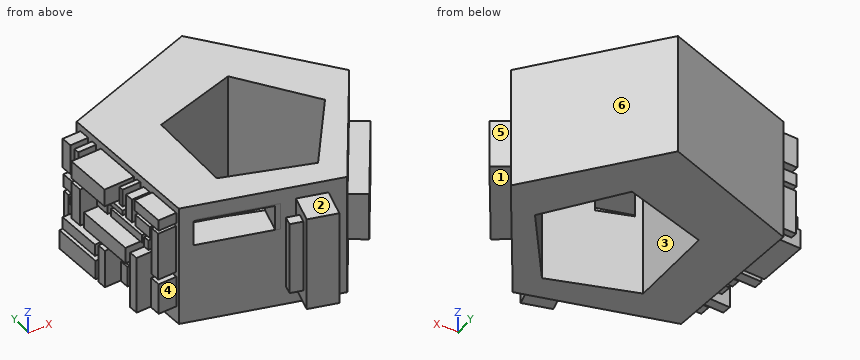
```python
from build123d import *

# Parameters (mm, degrees)
F1_DEPTH  = 25.4
F2_DEPTH  = 25.4
F3_W      = 42.2709332779
F3_H      = 19.9366761371
F4_DEPTH  = 7.62
F5_W      = 11.9896456599
F5_H      = 39.5106691867
F6_DEPTH  = 12.7
F7_W      = 31.212631613
F7_H      = 11.2281162292
F8_DEPTH  = 7.62
F9_W      = 29.9386493862
F9_H      = 10.5491885915
F10_DEPTH = 12.7
F11_W     = 4.0996596217
F11_H     = 30.3628398106
F12_DEPTH = 5.08
F13_W     = 20.0984636322
F13_H     = 7.4342815205
F13_W_2   = 5.3358711302
F13_H_2   = 15.8698209561
F13_W_3   = 25.2564756665
F13_H_3   = 6.7615092266
F13_W_4   = 3.9129797369
F13_H_4   = 16.0269849002
F13_W_5   = 19.5648819208
F13_H_5   = 4.9852463417
F13_W_6   = 21.8770895153
F13_H_6   = 8.1112636253
F13_W_7   = 3.8565089926
F13_H_7   = 24.0716314875
F14_DEPTH = 12.7
F15_W     = 2.3439750075
F15_H     = 14.3474126235
F15_W_2   = 10.4969404638
F15_H_2   = 5.3929993883
F15_W_3   = 4.6879537404
F15_H_3   = 12.7176120877
F15_W_4   = 2.7516260743
F15_H_4   = 18.800791353
F15_W_5   = 6.8281069398
F15_H_5   = 3.639341332
F15_W_6   = 10.8026759699
F15_H_6   = 4.3754521757
F15_W_7   = 4.6879523434
F15_H_7   = 8.343886584
F15_W_8   = 3.7707453594
F15_H_8   = 8.649148047
F15_W_9   = 6.2166322023
F15_H_9   = 3.6631692201
F15_W_10  = 14.7772468626
F15_H_10  = 2.1284492686
F15_W_11  = 18.8184157014
F15_H_11  = 3.3579049632
F15_W_12  = 3.6688325927
F15_H_12  = 10.0737148896
F15_W_13  = 1.9363295287
F15_H_13  = 7.4342815205
F15_W_14  = 14.4715099595
F15_H_14  = 4.57723625
F15_W_15  = 8.7644355372
F15_H_15  = 4.8842262477
F15_W_16  = 3.9745708928
F15_H_16  = 20.249187015
F15_W_17  = 2.5478007738
F15_H_17  = 4.1719428264
F15_W_18  = 4.586043302
F15_H_18  = 13.0246016197
F16_DEPTH = 7.62
F17_W     = 61.8985138723
F17_H     = 50.8
F17_W_2   = 21.8770895153
F17_H_2   = 8.1112636253
F17_W_3   = 2.7516260743
F17_H_3   = 18.800791353
F17_W_4   = 6.8281069398
F17_H_4   = 3.639341332
F17_W_5   = 19.5648819208
F17_H_5   = 4.9852463417
F17_W_6   = 3.7707453594
F17_H_6   = 8.649148047
F17_W_7   = 4.6879523434
F17_H_7   = 8.343886584
F17_W_8   = 3.9129797369
F17_H_8   = 16.0269849002
F17_W_9   = 10.8026759699
F17_H_9   = 4.3754521757
F17_W_10  = 3.8565089926
F17_H_10  = 24.0716314875
F17_W_11  = 4.586043302
F17_H_11  = 13.0246016197
F17_W_12  = 10.4969404638
F17_H_12  = 5.3929993883
F17_W_13  = 5.3358711302
F17_H_13  = 15.8698209561
F17_W_14  = 6.2166322023
F17_H_14  = 3.6631692201
F17_W_15  = 4.6879537404
F17_H_15  = 12.7176120877
F17_W_16  = 2.3439750075
F17_H_16  = 14.3474126235
F17_W_17  = 20.0984636322
F17_H_17  = 7.4342815205
F17_W_18  = 25.2564756665
F17_H_18  = 6.7615092266
F17_W_19  = 14.7772468626
F17_H_19  = 2.1284492686
F17_W_20  = 18.8184157014
F17_H_20  = 3.3579049632
F17_W_21  = 2.5478007738
F17_H_21  = 4.1719428264
F17_W_22  = 3.9745708928
F17_H_22  = 20.249187015
F17_W_23  = 1.9363295287
F17_W_24  = 3.6688325927
F17_H_23  = 10.0737148896
F17_W_25  = 8.7644355372
F17_H_24  = 4.8842262477
F17_W_26  = 14.4715099595
F17_H_25  = 4.57723625
F18_DEPTH = 5.08
F20_DEPTH = 76.2
F21_DEPTH = 5.08


with BuildPart() as f1:
    # F0 (on Top) → F1 (new body)
    with BuildSketch(Plane.XY):
        Polygon((-16.7726497146, -31.6705114622), (16.7726497146, 20.3500508744), (-22.335777472, 68.3287643065), (-80.051414149, 45.9606776074), (-76.6132121111, -15.842273668), align=None)
    extrude(amount=F1_DEPTH)

    # F2 (add): a face of the model
    f2_faces = [f1.faces().sort_by_distance(p)[0] for p in [
        (-35.8000807464, 17.4253415316, 0),
    ]]
    extrude(f2_faces, amount=F2_DEPTH)

    # F3 (on face) → F4 (join)
    with BuildSketch(Plane(origin=(2.5779849193, -1.6624056365, 0), x_dir=(0.5419403041, 0.8404169839, 0), z_dir=(0.8404169839, -0.5419403041, 0))):
        with Locations((-5.966336932, 1.3790032826)):
            Rectangle(F3_W, F3_H)
    extrude(amount=F4_DEPTH)

    # F5 (on face) → F6 (join)
    with BuildSketch(Plane(origin=(-8.9260455296, -33.7459919046, 0), x_dir=(0.9667528128, -0.2557127272, 0), z_dir=(-0.2557127272, -0.9667528128, 0))):
        with Locations((-20.9904853255, 0.3661895171)):
            Rectangle(F5_W, F5_H)
    extrude(amount=F6_DEPTH)

    # F7 (on face) → F8 (join)
    with BuildSketch(Plane(origin=(-8.9260455296, -33.7459919046, 0), x_dir=(0.9667528128, -0.2557127272, 0), z_dir=(-0.2557127272, -0.9667528128, 0))):
        with Locations((-48.2821147889, 13.5751133785)):
            Rectangle(F7_W, F7_H)
    extrude(amount=-F8_DEPTH)

    # F9 (on face) → F10 (cut)
    with BuildSketch(Plane(origin=(-8.9260455296, -33.7459919046, 0), x_dir=(0.9667528128, -0.2557127272, 0), z_dir=(-0.2557127272, -0.9667528128, 0))):
        with Locations((-49.556100741, 13.31924228)):
            Rectangle(F9_W, F9_H)
    extrude(amount=-F10_DEPTH, mode=Mode.SUBTRACT)

    # F11 (on face) → F12 (join)
    with BuildSketch(Plane(origin=(-26.0881225645, 6.9004867437, 0), x_dir=(-0.2557127272, -0.9667528128, 0), z_dir=(-0.9667528128, 0.2557127272, 0))):
        with Locations((41.5847562253, 1.0980186053)):
            Rectangle(F11_W, F11_H)
    extrude(amount=F12_DEPTH)

    # F13 (on face) → F14 (join)
    with BuildSketch(Plane(origin=(-77.2554477784, -4.2978503859, 0), x_dir=(0.055545793, -0.9984561407, 0), z_dir=(-0.9984561407, -0.055545793, 0))):
        with Locations((-25.5797388963, 18.8945052214)):
            Rectangle(F13_W, F13_H)
        with Locations((-32.961031422, 5.5121385958)):
            Rectangle(F13_W_2, F13_H_2)
        with Locations((-15.5305069638, 1.3388268417)):
            Rectangle(F13_W_3, F13_H_3)
        with Locations((-17.3091338947, -12.3113878071)):
            Rectangle(F13_W_4, F13_H_4)
        with Locations((-31.1824083328, -7.7815449331)):
            Rectangle(F13_W_5, F13_H_5)
        with Locations((-31.9827897474, -16.2692484446)):
            Rectangle(F13_W_6, F13_H_6)
        with Locations((1.9282544963, -7.5779159088)):
            Rectangle(F13_W_7, F13_H_7)
    extrude(amount=F14_DEPTH)

    # F15 (on face) → F16 (join)
    with BuildSketch(Plane(origin=(-77.2554477784, -4.2978503859, 0), x_dir=(0.055545793, -0.9984561407, 0), z_dir=(-0.9984561407, -0.055545793, 0))):
        with Locations((-39.761338383, 15.3379100375)):
            Rectangle(F15_W, F15_H)
        with Locations((-42.4110535532, 4.5519121923)):
            Rectangle(F15_W_2, F15_H_2)
        with Locations((-45.7231942564, 16.2528399378)):
            Rectangle(F15_W_3, F15_H_3)
        with Locations((-45.9779724479, -9.4003956765)):
            Rectangle(F15_W_4, F15_H_4)
        with Locations((-39.9651639163, -1.819670666)):
            Rectangle(F15_W_5, F15_H_5)
        with Locations((-7.5061791576, -6.2340861186)):
            Rectangle(F15_W_6, F15_H_6)
        with Locations((-4.7545537818, -13.407792896)):
            Rectangle(F15_W_7, F15_H_7)
        with Locations((-10.7164080255, -13.8656888157)):
            Rectangle(F15_W_8, F15_H_8)
        with Locations((-24.066885002, 8.0624492839)):
            Rectangle(F15_W_9, F15_H_9)
        with Locations((-19.1751066595, 12.3828244396)):
            Rectangle(F15_W_10, F15_H_10)
        with Locations((-9.4092078507, 8.2150814123)):
            Rectangle(F15_W_11, F15_H_11)
        with Locations((-7.9138264991, 16.7624759488)):
            Rectangle(F15_W_12, F15_H_12)
        with Locations((-12.7546479926, 18.8945052214)):
            Rectangle(F15_W_13, F15_H_13)
        with Locations((2.7869374026, 20.3230278566)):
            Rectangle(F15_W_14, F15_H_14)
        with Locations((0.3410479985, 13.9642218128)):
            Rectangle(F15_W_15, F15_H_15)
        with Locations((7.8315832652, 6.4852521755)):
            Rectangle(F15_W_16, F15_H_16)
        with Locations((2.5321574649, 7.8080624808)):
            Rectangle(F15_W_17, F15_H_17)
        with Locations((7.831583498, -11.9832272176)):
            Rectangle(F15_W_18, F15_H_18)
    extrude(amount=F16_DEPTH)

    # F17 (on face) → F18 (cut)
    with BuildSketch(Plane(origin=(-77.2554477784, -4.2978503859, 0), x_dir=(0.055545793, -0.9984561407, 0), z_dir=(-0.9984561407, -0.055545793, 0))):
        with Locations((-19.38698313, 0)):
            Rectangle(F17_W, F17_H)
        with Locations((-31.9827897474, -16.2692484446)):
            Rectangle(F17_W_2, F17_H_2, mode=Mode.SUBTRACT)
        with Locations((-45.9779724479, -9.4003956765)):
            Rectangle(F17_W_3, F17_H_3, mode=Mode.SUBTRACT)
        with Locations((-39.9651639163, -1.819670666)):
            Rectangle(F17_W_4, F17_H_4, mode=Mode.SUBTRACT)
        with Locations((-31.1824083328, -7.7815449331)):
            Rectangle(F17_W_5, F17_H_5, mode=Mode.SUBTRACT)
        with Locations((-10.7164080255, -13.8656888157)):
            Rectangle(F17_W_6, F17_H_6, mode=Mode.SUBTRACT)
        with Locations((-4.7545537818, -13.407792896)):
            Rectangle(F17_W_7, F17_H_7, mode=Mode.SUBTRACT)
        with Locations((-17.3091338947, -12.3113878071)):
            Rectangle(F17_W_8, F17_H_8, mode=Mode.SUBTRACT)
        with Locations((-7.5061791576, -6.2340861186)):
            Rectangle(F17_W_9, F17_H_9, mode=Mode.SUBTRACT)
        with Locations((1.9282544963, -7.5779159088)):
            Rectangle(F17_W_10, F17_H_10, mode=Mode.SUBTRACT)
        with Locations((7.831583498, -11.9832272176)):
            Rectangle(F17_W_11, F17_H_11, mode=Mode.SUBTRACT)
        with Locations((-42.4110535532, 4.5519121923)):
            Rectangle(F17_W_12, F17_H_12, mode=Mode.SUBTRACT)
        with Locations((-32.961031422, 5.5121385958)):
            Rectangle(F17_W_13, F17_H_13, mode=Mode.SUBTRACT)
        with Locations((-24.066885002, 8.0624492839)):
            Rectangle(F17_W_14, F17_H_14, mode=Mode.SUBTRACT)
        with Locations((-45.7231942564, 16.2528399378)):
            Rectangle(F17_W_15, F17_H_15, mode=Mode.SUBTRACT)
        with Locations((-39.761338383, 15.3379100375)):
            Rectangle(F17_W_16, F17_H_16, mode=Mode.SUBTRACT)
        with Locations((-25.5797388963, 18.8945052214)):
            Rectangle(F17_W_17, F17_H_17, mode=Mode.SUBTRACT)
        with Locations((-15.5305069638, 1.3388268417)):
            Rectangle(F17_W_18, F17_H_18, mode=Mode.SUBTRACT)
        with Locations((-19.1751066595, 12.3828244396)):
            Rectangle(F17_W_19, F17_H_19, mode=Mode.SUBTRACT)
        with Locations((-9.4092078507, 8.2150814123)):
            Rectangle(F17_W_20, F17_H_20, mode=Mode.SUBTRACT)
        with Locations((2.5321574649, 7.8080624808)):
            Rectangle(F17_W_21, F17_H_21, mode=Mode.SUBTRACT)
        with Locations((7.8315832652, 6.4852521755)):
            Rectangle(F17_W_22, F17_H_22, mode=Mode.SUBTRACT)
        with Locations((-12.7546479926, 18.8945052214)):
            Rectangle(F17_W_23, F17_H_17, mode=Mode.SUBTRACT)
        with Locations((-7.9138264991, 16.7624759488)):
            Rectangle(F17_W_24, F17_H_23, mode=Mode.SUBTRACT)
        with Locations((0.3410479985, 13.9642218128)):
            Rectangle(F17_W_25, F17_H_24, mode=Mode.SUBTRACT)
        with Locations((2.7869374026, 20.3230278566)):
            Rectangle(F17_W_26, F17_H_25, mode=Mode.SUBTRACT)
    extrude(amount=-F18_DEPTH, mode=Mode.SUBTRACT)

    # F19 (on face) → F20 (cut)
    with BuildSketch(Plane.XY.offset(25.4)):
        Polygon((-55.9489503503, 28.6254710477), (-55.9489503503, -8.0040893477), (-21.1121682472, -19.3232460063), (0.4181471511, 10.31069085), (-21.1121682472, 39.9446277064), align=None)
    extrude(amount=-F20_DEPTH, mode=Mode.SUBTRACT)

    # F21 (add): a face of the model
    f21_faces = [f1.faces().sort_by_distance(p)[0] for p in [
        (-71.5855334196, -14.7605835197, 0),
    ]]
    extrude(f21_faces, amount=F21_DEPTH)


solid = f1.part
```
Here's how the part is built. I have some questions about the finished solid (model axes, mm). Face numbers are marked on the shaded views. A direction names the side the tool comes from. Give positions to 0.01 mm unless a question says otherwise; leave off trailing zeros. Write each loop counter-clockwise with the first axis right and the second up, starting at its lowest first coordinate (ties: lowest second). Pieces come first, ordered by that corner, then holes. Notation, with made-up numbers: (68.25, 25) -> (79.25, 25) arc R25 cw to (79.25, 61) -> close; hole circle Ø8 at (43.25, 31). An arc over 180 degrees is marked (long way). Use one line per item in the form item = value.
1) On a 3-axis mill with a long thin cutter (end or side, diameter ignored), from which of +Z, -Z, +X, -X, +Y, -Y can I reach the whole of each face in a straight line? I mean the marked faces 1, 2 and 3. Say none if no direction works.
Verdict:
face_1 = -Z, +X, -Y
face_2 = +Z, -X, -Y
face_3 = +Z, -Z
2) Suppose I cut it at D-D (y = 48). Please give me the cut outline in (x, z), and give its area (3 significant figures).
Verdict:
outline = (-74.79, -25.4) -> (-5.77, -25.4) -> (-5.77, 25.4) -> (-74.79, 25.4) -> close
area = 3,510 mm2
3) If I drill on L1, parallel to Z at x = -84, y = 12.5; L2, parallel to Z at x = -80, y = 22.5; L3, parallel to Y at x = -39, z = -6, over which ranges is the centre line in solid material (lowest first)? Write a range as [from, to].
Verdict:
L1 = [-20.32, -4.3], [-2.04, 4.72], [6.54, 9.89], [11.32, 13.45], [15.18, 22.61]
L2 = [-20.32, -12.21], [-10.27, -5.29], [-2.04, 4.72], [6.23, 9.89], [15.18, 22.61]
L3 = [-34.82, -30.58], [-25.79, -13.51], [34.13, 61.87]
4) Suppose I cut it at B-B (z = -22). Please give me the cut outline in (x, y).
Verdict:
outline = (-80.05, 45.96) -> (-76.61, -15.84) -> (-16.77, -31.67) -> (16.77, 20.35) -> (-22.34, 68.33) -> close; hole (-55.95, -8) -> (-21.11, -19.32) -> (0.42, 10.31) -> (-21.11, 39.94) -> (-55.95, 28.63) -> close
5) Suppose I cut it at A-A (x = -30.5). Please give me the cut outline in (y, z), and give its area (3 significant figures).
Verdict:
outline = (-41.18, -19.39) -> (-28.04, -19.39) -> (-28.04, -25.4) -> (-16.27, -25.4) -> (-16.27, 25.4) -> (-28.04, 25.4) -> (-28.04, 20.12) -> (-41.18, 20.12) -> close; (36.89, -25.4) -> (65.16, -25.4) -> (65.16, 25.4) -> (36.89, 25.4) -> close
area = 2,550 mm2
6) I'm going to push flat-ended pins straight in: pin 1 (6 mm diameter, centred on y = 0.5, z = -7.5, fed in from +X); pin 2 (3 mm diameter, centred on x = -38.5, z = 18, fed in from -Y); pin 3 (10 mm diameter, centred on x = -46, z = -12, fed in from -Y). Where does each tip first touch, or does it pass through?
Verdict:
pin_1 = 14.97
pin_2 = -39.46
pin_3 = -34.29
7) Suppose I cut it at C-C (x = 3). Please give me the cut outline in (y, z), and give its area (3 significant figures).
Verdict:
outline = (-15.07, -8.59) -> (-1.01, -8.59) -> (-1.01, -25.4) -> (37.25, -25.4) -> (37.25, 25.4) -> (-1.01, 25.4) -> (-1.01, 11.35) -> (-15.07, 11.35) -> close
area = 2,220 mm2
8) We'd pull the mould along Y, two halves only. Please class the marked faces 4, 5 and 6: +Y half, -Y half, draft (parallel to the pull), parting line (faces both ways), or undercut.
Verdict:
face_4 = -Y half
face_5 = undercut
face_6 = +Y half
